Drawing for the job (mm, zero at the part's lowest x, y, z). A direction names the side the tool comes from. Round coordinates to 2 decimals unless told otherwise and drop trailing zeros. Loops run counter-clockwise (first coordinate to the right, second up) from the corner with the lowest first, then second, coordinate; pieces in that order, holes last. Notation, with made-up numbers: M 11,20.25 L 28,20.25 A16 cw 28,29.25 Z; hole C -32.75,3 d10. An arc over 180 degrees is marked long. Answer in a Markdown table with one row per item.
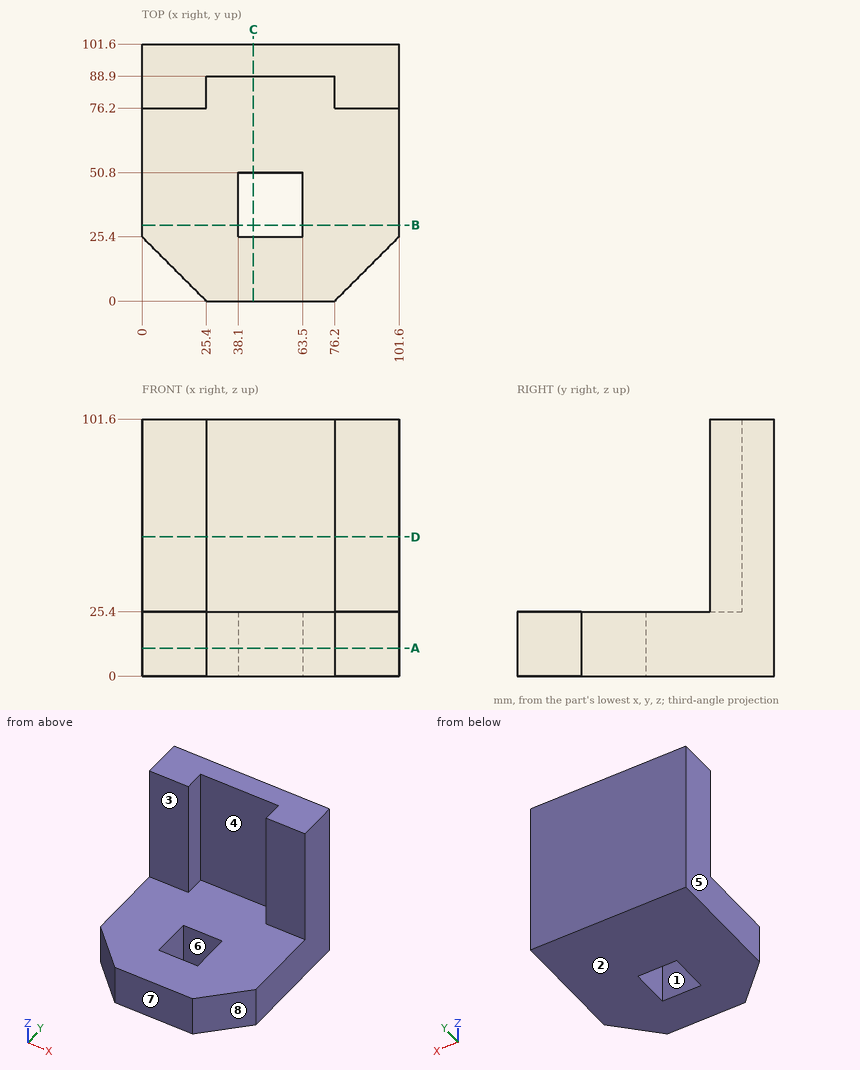
1. Wall check: probe 1 along X at (y, z) = (31.5, 13.5); probe 2 along Y at (x, z) = (46.5, 8.5); probe 3 along Y at (x, z) = (42.5, 72). Give the ranges that are in metal, low to high.
Verdict:
| item | result |
|---|---|
| probe 1 | x = 0 to 38.1, 63.5 to 101.6 |
| probe 2 | y = 0 to 25.4, 50.8 to 101.6 |
| probe 3 | y = 88.9 to 101.6 |
2. Tool access for the marked faces 1, 2, 3 and 4: list every direction of +Z, -Z, +X, -X, +Y, -Y with a clear straight run to the whole face (end or side of a thin tool).
Verdict:
| item | result |
|---|---|
| face 1 | +Z, -Z |
| face 2 | -Z, +X, -X, +Y, -Y |
| face 3 | +Z, +X, -X, -Y |
| face 4 | +Z, -Y |
3. Saw through at A-A (z = 11). Write the cut outline in (x, y).
Verdict:
| item | result |
|---|---|
| outline | M 0,25.4 L 25.4,0 L 76.2,0 L 101.6,25.4 L 101.6,101.6 L 0,101.6 Z; hole M 38.1,25.4 L 63.5,25.4 L 63.5,50.8 L 38.1,50.8 Z |
4. Saw through at D-D (z = 55). Write the cut outline in (x, y), and give its area (3 significant figures).
Verdict:
| item | result |
|---|---|
| outline | M 0,76.2 L 25.4,76.2 L 25.4,88.9 L 76.2,88.9 L 76.2,76.2 L 101.6,76.2 L 101.6,101.6 L 0,101.6 Z |
| area | 1,940 mm² |
5. Mould opens along X. For the marked faces 5, 6, 7 and 8 say: +X half, -X half, draft (parallel to the pull), parting line (faces both ways), or undercut.
Verdict:
| item | result |
|---|---|
| face 5 | -X half |
| face 6 | undercut |
| face 7 | draft |
| face 8 | +X half |
6. Pin check, flat tips, straight feed: pin 1 (4 mm diameter, centred on x = 26.5, z = 80.5, fed in from -Y); pin 2 (4 mm diameter, centred on x = 79, y = 59, fed in from +Z); pin 3 (2 mm diameter, centred on x = 59, z = 50.5, fed in from -Y). Stop position of each tip, or through.
Verdict:
| item | result |
|---|---|
| pin 1 | stops at y = 76.2 |
| pin 2 | stops at z = 25.4 |
| pin 3 | stops at y = 88.9 |
7. Saw through at C-C (x = 44). Write the cut outline in (y, z), and give its area (3 significant figures).
Verdict:
| item | result |
|---|---|
| outline | M 0,0 L 25.4,0 L 25.4,25.4 L 0,25.4 Z; M 50.8,0 L 101.6,0 L 101.6,101.6 L 88.9,101.6 L 88.9,25.4 L 50.8,25.4 Z |
| area | 2,900 mm² |
8. Saw through at B-B (y = 30). Write the cut outline in (x, z), and give its area (3 significant figures).
Verdict:
| item | result |
|---|---|
| outline | M 0,0 L 38.1,0 L 38.1,25.4 L 0,25.4 Z; M 63.5,0 L 101.6,0 L 101.6,25.4 L 63.5,25.4 Z |
| area | 1,940 mm² |
